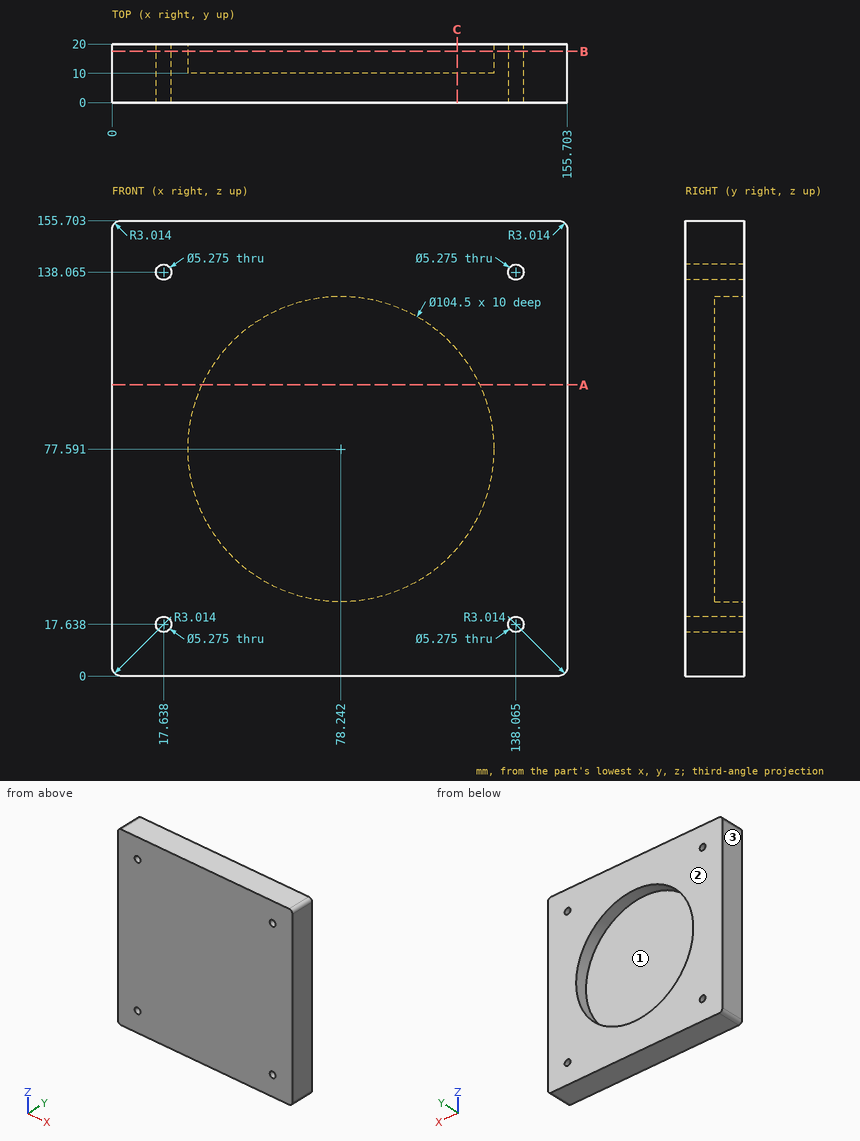
Source: three-view drawing plus pictorial views. Frame: mm from the lowest corner of the part. Give positions to 0.01 mm unless a question says otherwise; leave off trailing zeros. Order: outer loops, then holes, each group sorted by start corner. A loop starts at its lowest first (then second) coordinate and runs counter-clockwise, first axis right, second up. Notation, with made-up numbers: (-15.5, -24) -> (18.5, -24) arc R21 cw to (18.5, -4) -> close; hole circle Ø7 at (53, 75.25). An arc over 180 degrees is marked (long way). Put each result on its own line as item: value.
Q1. Material intervals for L1, parallel to Y at x = 113, z = 57; L2, parallel to Z at x = 97, y = 14.25 (1 decimal); L3, parallel to X at y = 16, z = 81.5 (1 decimal), sorted ascending.
Here are the results:
L1: y = 0 to 10
L2: z = 0 to 28.8, 126.4 to 155.7
L3: x = 0 to 26.1, 130.3 to 155.7
Q2. Pin query (flat end, axial travel): pin 1 (4 mm diameter, centred on x = 56.5, y = 10.5, fed in from -Z); pin 2 (10 mm diameter, centred on x = 42.5, z = 92, fed in from +Y); pin 3 (4 mm diameter, centred on x = 138.07, z = 138.07, fed in from +Y). Return the tip coordinate at first contact, or that it passes through.
Here are the results:
pin 1: stops at z = 0
pin 2: stops at y = 10
pin 3: passes through
Q3. Section C-C, the plane x = 118. Return loops of the section in (y, z), then the cut area to 3 significant figures.
Here are the results:
outline: (0, 0) -> (20, 0) -> (20, 43.69) -> (10, 43.69) -> (10, 111.49) -> (20, 111.49) -> (20, 155.7) -> (0, 155.7) -> close
area: 2,440 mm^2
Q4. Section B-B, the plane y = 17.5. Count the separate pieces of the cut face and the enclosed holes in it, then the cut area to 3 significant figures.
Here are the results:
separate pieces: 1
enclosed holes: 5
area: 15,600 mm^2
Q5. Draft query along X for the marked faces 1, 2 and 3. Return one class per face: released by +X, released by -X, zero draft, split by the parting line, or undercut.
Here are the results:
face 1: undercut
face 2: zero draft
face 3: released by -X
Q6. Section A-A, the plane z = 99.5. Return loops of the section in (x, y), then the cut area to 3 significant figures.
Here are the results:
outline: (0, 0) -> (155.7, 0) -> (155.7, 20) -> (125.68, 20) -> (125.68, 10) -> (30.81, 10) -> (30.81, 20) -> (0, 20) -> close
area: 2,170 mm^2
